Can you work these out from the model? Positions are in its coordinate system, mm. A direction names the side the tool comes from. Coordinates: 2 decimals unless noted, no trailing zeros. Order: outer loops, then holes, each group sorted by start corner. A loop starts at its lowest first (then second) coordinate and runs counter-clockwise, first axis right, second up. Notation, with made-up numbers: (60, 39) -> (86, 39) arc R26 ccw to (86, 73) -> close; hole circle Ø9 at (54, -35.5). An arc over 180 degrees is marked (long way). Answer as CSV lines item,"result".
from build123d import *

# Parameters (mm, degrees)
SKETCH1_W           = 8
SKETCH1_H           = 5
BOSS_EXTRUDE1_DEPTH = 0.5
SKETCH2_W           = 8
SKETCH2_H           = 1
BOSS_EXTRUDE2_DEPTH = 0.5
SKETCH3_R           = 2
BOSS_EXTRUDE3_DEPTH = 1
SWEEP5_PROFILE_R    = 2


with BuildPart() as part:
    # Sketch1 → Boss-Extrude1 (new body)
    with BuildSketch(Plane(origin=(0, 0, 0), x_dir=(1, 0, 0), z_dir=(0, 1, 0))):
        with Locations((4, 2.5)):
            Rectangle(SKETCH1_W, SKETCH1_H)
    extrude(amount=BOSS_EXTRUDE1_DEPTH)

    # Sketch2 → Boss-Extrude2 (add)
    with BuildSketch(Plane.XZ):
        with Locations((4, -0.5)):
            Rectangle(SKETCH2_W, SKETCH2_H)
        with Locations((4, -4.5)):
            Rectangle(SKETCH2_W, SKETCH2_H)
    extrude(amount=BOSS_EXTRUDE2_DEPTH)

    # Sketch3 → Boss-Extrude3 (add)
    with BuildSketch(Plane(origin=(0, 0.5, 0), x_dir=(1, 0, 0), z_dir=(0, 1, 0))):
        with Locations((4, 2.5)):
            Circle(SKETCH3_R)
    extrude(amount=BOSS_EXTRUDE3_DEPTH)

    # Sweep5: sweep along a path in Sketch6
    with BuildLine(Plane.XY.offset(-2.5)) as sweep5_path:
        Line((4, 1.5), (4, 6.626951227))
        ThreePointArc((4, 6.626951227), (-1.083608385, 19.949911153), (-13.750126119, 26.5))
    # Sweep5 profile (on start of the path) → Sweep5 (sweep)
    with BuildSketch(Plane(origin=(4, 1.5, -2.5), x_dir=(1, 0, 0), z_dir=(0, 1, 0))):
        Circle(SWEEP5_PROFILE_R)
    sweep(path=sweep5_path.line)


solid = part.part
Q1. For P1, Ø1.1, axis at y = 0, z = -2, coming from the -X side; P2, Ø0.9, axis at x = 4, z = -2, coming from the -Y side; P3, Ø2, axis at y = 13, z = -1, coming from the -X side; P4, Ø0.6, axis at x = 4.5, y = 0, coming from the +Z side, each with a flat end and sliding along its axis, tell me the tip position at first contact or that it passes through.
Solution:
P1,"x = 0"
P2,"y = 0"
P3,"x = 0.73"
P4,"z = 0"
Q2. Imagine slicing it at B-B (y = 6). List the corners of the cut face in (x, z) for me, and give its area (3 significant figures).
Solution:
outline,"circle Ø4 at (4, -2.5)"
area,"12.6 mm2"
Q3. We'd pull the mould along Z, two halves only. Please class faces 4 (the flat face through (4, 0, -5)), 5 (the flat face through (8, 0.2, -2.5)), 6 (the flat face through (4, 0, -3)), 7 (the flat face through (4, 0, 0)): pulls with the +Z half, pulls with the -Z half, needs draft (parallel to the pull), parting line crosses it, or undercut.
Solution:
face 4,"pulls with the -Z half"
face 5,"needs draft"
face 6,"undercut"
face 7,"pulls with the +Z half"
Q4. Imagine slicing it at A-A (z = -2.5). List the corners of the cut face in (x, y) for me, and give its area (3 significant figures).
Solution:
outline,"(-13.98, 24.51) arc R18 cw to (2, 6.63) -> (2, 0.5) -> (0, 0.5) -> (0, 0) -> (8, 0) -> (8, 0.5) -> (6, 0.5) -> (6, 6.63) arc R22 ccw to (-13.53, 28.49) -> close"
area,"145 mm2"
Q5. Which directions (+Z, -Z, +X, -X, +Y, -Y) give clear straight access to the entire face, cutting with the end or side of a thin tool? Please do faces 1 (the flat face through (6, 0.5, -4)), 2 (the flat face through (0, 0.2, -2.5)), 3 (the flat face through (3.9, -0.5, -4.5)).
Solution:
face 1,"none"
face 2,"+Z, -Z, -X, -Y"
face 3,"+Z, -Z, +X, -X, -Y"
Q6. If I drill on line 1 (Y direction, x = -2.5, z = -2.3); line 2 (Y direction, x = -7.75, z = -4.2); line 3 (X direction, y = 21.25, z = -1.2), over which ranges is the centre line in solid material (lowest first)?
Solution:
line 1,"18.55 to 23.99"
line 2,"23.68 to 26"
line 3,"-4.7 to -0.21"
